Can you work these out from the model? Positions are in its coordinate system, mm. A direction names the side the tool comes from. Round coordinates to 2 decimals unless told otherwise and drop trailing zeros. Order: outer loops, then holes, each group sorted by start corner. A loop starts at its lowest first (then second) coordinate and runs counter-clockwise, first axis right, second up. Notation, with made-up numbers: (62, -11) -> (75, -11) arc R20 ccw to (75, -3) -> close; hole circle Ø2 at (10.25, -14). An arc over 180 degrees is marked (long way). One line per item, written item: value.
```python
from build123d import *

# Parameters (mm, degrees)
SKETCH007_W   = 13.5
SKETCH007_H   = 13.5
PAD005_DEPTH  = 3.5
SKETCH008_R   = 3.375
SKETCH008_R_2 = 1.35
PAD006_DEPTH  = 8
SKETCH009_W   = 13.5
SKETCH009_H   = 16.91
SKETCH009_R   = 1.5
PAD007_DEPTH  = 3


with BuildPart() as part:
    # Sketch007 → Pad005 (new body)
    with BuildSketch(Plane.XY):
        with Locations((6.75, 6.75)):
            Rectangle(SKETCH007_W, SKETCH007_H)
    extrude(amount=PAD005_DEPTH)

    # Sketch008 (on Face6 of Pad005) → Pad006 (join)
    with BuildSketch(Plane.XY.offset(3.5)):
        with Locations((6.75, 6.75)):
            Circle(SKETCH008_R)
        with Locations((6.75, 6.75)):
            Circle(SKETCH008_R_2, mode=Mode.SUBTRACT)
    extrude(amount=PAD006_DEPTH)

    # Sketch009 (on Face2 of Pad006) → Pad007 (join)
    with BuildSketch(Plane(origin=(0, 0, 0), x_dir=(0, -1, 0), z_dir=(-1, 0, 0))):
        with Locations((-6.75, 8.455)):
            Rectangle(SKETCH009_W, SKETCH009_H)
        with Locations((-6.75, 9.91)):
            Circle(SKETCH009_R, mode=Mode.SUBTRACT)
    extrude(amount=PAD007_DEPTH)


solid = part.part
```
Q1. We'd pull the mould along Y, two halves only. Please class faces 1 (the face through (9.87, 5.46, 7.44)), 2 (the face through (2, 0, 3)), 3 (the face through (7.476, 7.888, 7.444)), 4 (the face through (5, 10, 3.5)): released by +Y, released by -Y, zero draft, split by the parting line, or undercut.
Answers below:
face 1: split by the parting line
face 2: released by -Y
face 3: undercut
face 4: zero draft
Q2. On a 3-axis mill with a long thin cutter (end or side, diameter ignored), from which of +Z, -Z, +X, -X, +Y, -Y can I reach the whole of each face in a straight line? I mean faces 5 (the face through (7, 7, 3.5)), 6 (the face through (-1.48, 7.94, 9)), 7 (the face through (0, 7, 12)). Say none if no direction works.
Answers below:
face 5: +Z
face 6: -X
face 7: +Z, +Y, -Y
Q3. I want a section at A-A on z = 9.91. List the corners of the cut face in (x, y) for me (3 decimals), plus the area to 3 significant figures.
Answers below:
outline: (-3, 0) -> (0, 0) -> (0, 5.25) -> (-3, 5.25) -> close; (-3, 8.25) -> (0, 8.25) -> (0, 13.5) -> (-3, 13.5) -> close; circle Ø6.75 at (6.75, 6.75); hole circle Ø2.7 at (6.75, 6.75)
area: 61.6 mm^2
Q4. I want a section at D-D on x = 6.75. List the corners of the cut face in (y, z) for me (3 decimals), plus the area to 4 significant figures.
Answers below:
outline: (0, 0) -> (13.5, 0) -> (13.5, 3.5) -> (10.125, 3.5) -> (10.125, 11.5) -> (8.1, 11.5) -> (8.1, 3.5) -> (5.4, 3.5) -> (5.4, 11.5) -> (3.375, 11.5) -> (3.375, 3.5) -> (0, 3.5) -> close
area: 79.65 mm^2
Q5. Will these pins go through, and if not, where does the flat tip stop? pin 1 Ø4 at (y, z) = (5.5, 12.5) entering from +X (3 decimals); pin 2 Ø2 at (x, y) = (7.5, 8) entering from +Z; pin 3 Ø5 at (x, z) = (9, 11) entering from +Y (3 decimals).
Answers below:
pin 1: x = 10.125
pin 2: z = 11.5
pin 3: y = 10.125
Q6. I want a section at B-B on y = 6.75. List the corners of the cut face in (x, z) for me (3 decimals), plus the area to 3 significant figures.
Answers below:
outline: (-3, 0) -> (13.5, 0) -> (13.5, 3.5) -> (10.125, 3.5) -> (10.125, 11.5) -> (8.1, 11.5) -> (8.1, 3.5) -> (5.4, 3.5) -> (5.4, 11.5) -> (3.375, 11.5) -> (3.375, 3.5) -> (0, 3.5) -> (0, 8.41) -> (-3, 8.41) -> close; (-3, 11.41) -> (0, 11.41) -> (0, 16.91) -> (-3, 16.91) -> close
area: 121 mm^2
Q7. Please list where these lines run through material, in increasing order: line 1 along Y through (x, z) = (6.75, 7.5) (3 decimals); line 2 along X through (y, z) = (6, 3.75); line 3 along Z through (x, y) = (-2.3, 6.75).
Answers below:
line 1: 3.375 to 5.4, 8.1 to 10.125
line 2: -3 to 0, 3.46 to 5.63, 7.87 to 10.04
line 3: 0 to 8.41, 11.41 to 16.91
Q8. I want a section at C-C on z = 4.5. List the corners of the cut face in (x, y) for me (3 decimals).
Answers below:
outline: (-3, 0) -> (0, 0) -> (0, 13.5) -> (-3, 13.5) -> close; circle Ø6.75 at (6.75, 6.75); hole circle Ø2.7 at (6.75, 6.75)
